Geometry: see drawing. Coordinates: mm, zero at the bounding-box minimum. A direction names the side the tool comes from. Round coordinates to 2 decimals unless told otherwise and drop trailing zeros. Loops run counter-clockwise (first coordinate to the right, second up) from the corner with the lowest first, then second, coordinate; pieces in that order, holes last.
(1) Section A-A, the plane y = 10. Return the cut outline in (x, z).
(2) Material intervals for probe 1 along Z at (x, y) = (70.5, 16.75); probe 2 along X at (y, z) = (13, 17), sorted ascending.
(3) First-contact query: pin 1 Ø6 at (x, z) = (34, 28) entering from -Y (3 decimals). Flat tip, straight axial feed; report the tip coordinate or a pass-through.
(4) Section B-B, the plane z = 140.5. Return the cut outline in (x, y) (3 decimals).
(5) Mould query, pull axis X, two halves, no side actions, for the marked faces 3, 4 and 5. Classes: pulls with the +X half, pulls with the -X half, needs draft (parallel to the pull), parting line crosses it, or undercut.
(6) Section D-D, the plane z = 33. Return the cut outline in (x, y) (3 decimals).
(7) Section C-C, the plane x = 16.5. Return the cut outline in (y, z) (3 decimals), plus the area to 3 significant figures.
(8) Set-up query: the marked faces 1 and 2. Return all of +Z, -Z, +X, -X, +Y, -Y with unobstructed straight access to the full face (end or side cutting, diameter ignored); none if empty.
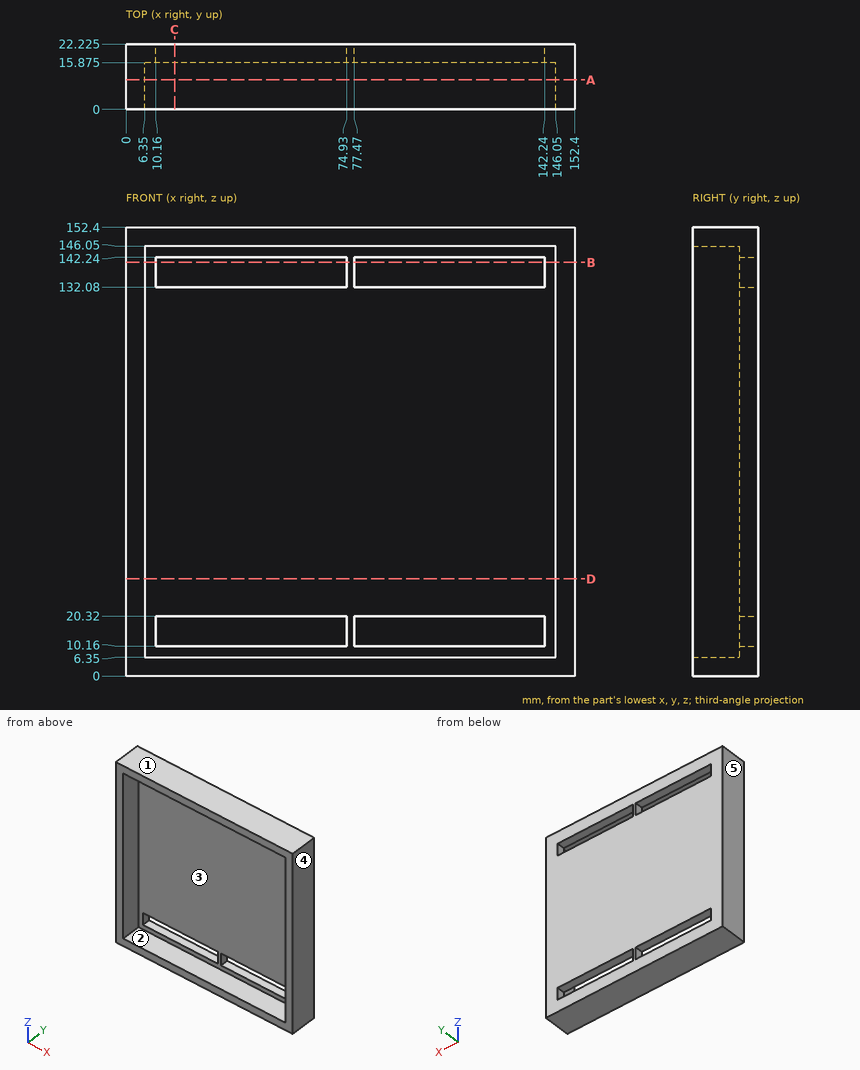
Output values:
1. outline: (0, 0) - (152.4, 0) - (152.4, 152.4) - (0, 152.4) - close; hole (6.35, 6.35) - (146.05, 6.35) - (146.05, 146.05) - (6.35, 146.05) - close
2. probe 1: z = 0 to 10.16, 20.32 to 132.08, 142.24 to 152.4
2. probe 2: x = 0 to 6.35, 146.05 to 152.4
3. pin 1: stops at y = 15.875
4. outline: (0, 0) - (6.35, 0) - (6.35, 15.875) - (10.16, 15.875) - (10.16, 22.225) - (0, 22.225) - close; (74.93, 15.875) - (77.47, 15.875) - (77.47, 22.225) - (74.93, 22.225) - close; (142.24, 15.875) - (146.05, 15.875) - (146.05, 0) - (152.4, 0) - (152.4, 22.225) - (142.24, 22.225) - close
5. face 3: undercut
5. face 4: pulls with the +X half
5. face 5: pulls with the -X half
6. outline: (0, 0) - (6.35, 0) - (6.35, 15.875) - (146.05, 15.875) - (146.05, 0) - (152.4, 0) - (152.4, 22.225) - (0, 22.225) - close
7. outline: (0, 0) - (22.225, 0) - (22.225, 10.16) - (15.875, 10.16) - (15.875, 6.35) - (0, 6.35) - close; (0, 146.05) - (15.875, 146.05) - (15.875, 142.24) - (22.225, 142.24) - (22.225, 152.4) - (0, 152.4) - close; (15.875, 20.32) - (22.225, 20.32) - (22.225, 132.08) - (15.875, 132.08) - close
7. area: 1,040 mm2
8. face 1: +Z, +X, -X, +Y, -Y
8. face 2: -Y
